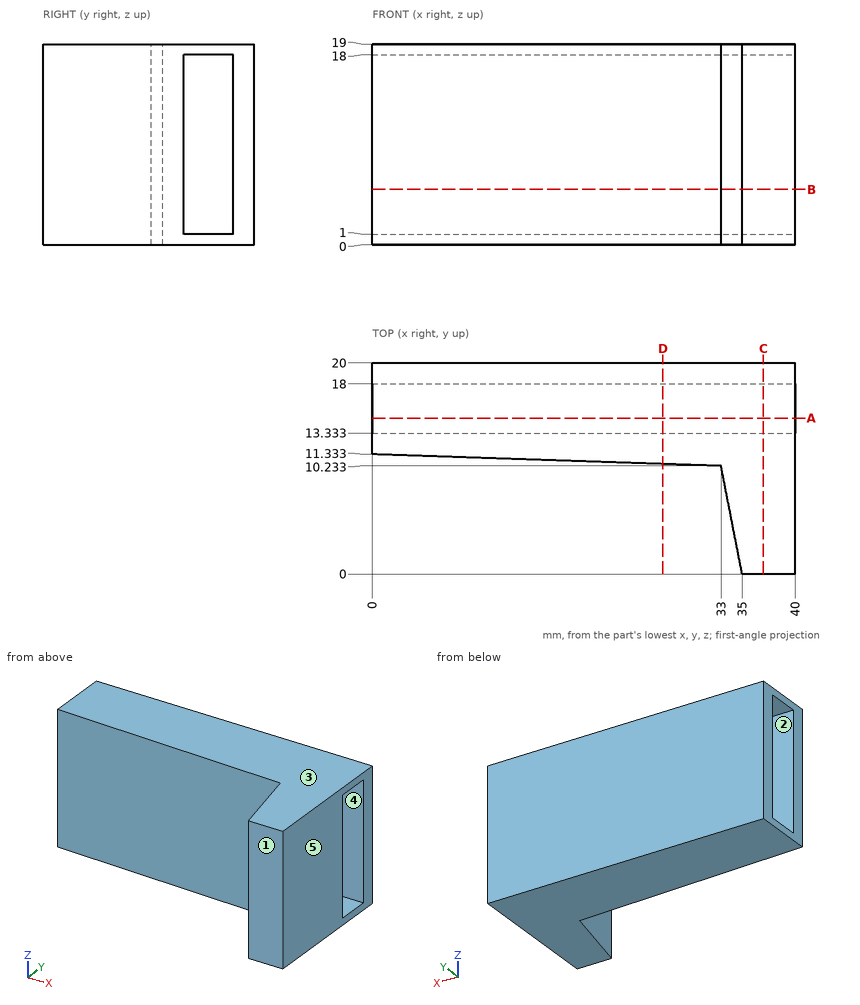
Study the drawing (mm; zero at the part's minimum x, y, z) and answer. A direction names the side the tool comes from. Round coordinates to 2 decimals unless told otherwise and drop trailing zeros. Loops run counter-clockwise (first coordinate to the right, second up) from the corner with the lowest first, then second, coordinate; pieces in that order, holes last. Notation, with made-up numbers: (89.5, 82) -> (117.5, 82) arc R11 cw to (117.5, 94) -> close; hole circle Ø11 at (43, -20). An arc over 180 degrees is marked (long way). Write each question's results on one line, items separated by ' | '. Start each with the question number.
1. A tool of negligible diameter and unlimited length cuts with its end or side. For the marked faces 1 and 2, from which of +Z, -Z, +X, -X, +Y, -Y can it reach the whole face along a straight path? Write none if from no direction.
2. Section A-A (y = 14.75) is taken. Determine the outline of the cut face in (x, z).
3. Section C-C (x = 37) is taken. Determine the outline of the cut face in (y, z), plus the area to 3 significant figures.
4. For a pull along Z with two mould halves and no side action, classify the marked faces 3, 4 and 5 as +Z half, -Z half, draft (parallel to the pull), parting line (faces both ways), or undercut.
5. Given pin 1 Ø3 at (x, y) = (32.5, 3) entering from -Z, flat-ended and moving along its own axis, determine where the tip first touches the part or whether it passes through.
6. Section D-D (x = 27.5) is taken. Determine the outline of the cut face in (y, z), plus the area to 3 significant figures.
7. Section B-B (z = 5.25) is taken. Determine the outline of the cut face in (x, y).
8. Find the intervals of material crossed by probe 1 along Z at (x, y) = (33, 13.5); probe 2 along Y at (x, z) = (25, 8); probe 3 along Y at (x, z) = (27.5, 11.5), in increasing order. Write a range as from..to.
Evaluation:
1) face 1: +Z, -Z, +X, -X, -Y | face 2: +X, -X
2) outline: (0, 0) -> (40, 0) -> (40, 1) -> (0, 1) -> close; (0, 18) -> (40, 18) -> (40, 19) -> (0, 19) -> close
3) outline: (0, 0) -> (20, 0) -> (20, 19) -> (0, 19) -> close; hole (13.33, 1) -> (18, 1) -> (18, 18) -> (13.33, 18) -> close | area: 301 mm2
4) face 3: +Z half | face 4: undercut | face 5: draft
5) pin 1: passes through
6) outline: (10.42, 0) -> (20, 0) -> (20, 19) -> (10.42, 19) -> close; hole (13.33, 1) -> (18, 1) -> (18, 18) -> (13.33, 18) -> close | area: 103 mm2
7) outline: (0, 11.33) -> (33, 10.23) -> (35, 0) -> (40, 0) -> (40, 13.33) -> (0, 13.33) -> close; (0, 18) -> (40, 18) -> (40, 20) -> (0, 20) -> close
8) probe 1: z = 0..1, 18..19 | probe 2: y = 10.5..13.33, 18..20 | probe 3: y = 10.42..13.33, 18..20
